The model under review builds one solid part; all positions refer to its coordinate system, in mm. Face numbers are marked on the shaded views. A direction names the side the tool comes from. Round coordinates to 2 decimals unless told otherwise and drop trailing zeros. Write each loop counter-clockwise with the first axis right and the second up, starting at its lowest first coordinate (ties: lowest second). Pieces come first, ordered by that corner, then holes. Notation, with made-up numbers: (-29, 80.5) -> (-2, 80.5) arc R32 ccw to (-2, 115.5) -> close; hole circle Ø11 at (68.5, 60). An arc over 180 degrees is marked (long way). Answer as a JSON object with one key per item and string values. Group by question number.
1) We need section D-D, the plane z = -6. Write out the cut boundary in (x, y), then the cut area to 3 significant figures.
2) We need section A-A, the plane x = 0. Write out the cut boundary in (y, z).
3) Mouldability with a two-part tool opening along Y and no side actions: class the marked faces 1, 2 and 3 as pulls with the +Y half, pulls with the -Y half, needs draft (parallel to the pull), parting line crosses it, or undercut.
4) To check wall thickness, follow probe 1 along X at (y, z) = (-1, -4.5); probe 2 along X at (y, z) = (-0.5, -2); probe 3 along Y at (x, z) = (1, -4.75). State the ranges of each line that lie inside material, in increasing order. Write a range as [from, to].
5) We need section B-B, the plane z = -12.5. Write out the cut boundary in (x, y), then the cut area to 3 significant figures.
6) We need section C-C, the plane z = -8.75. Write out the cut boundary in (x, y), then the cut area to 3 significant figures.
7) Machinability: for the marked faces 4, 5 and 6, which of the approach directions +Z, -Z, +X, -X, +Y, -Y give a long, thin tool a straight path to every point of the face, cutting with its end or side? Answer none if there is none.
8) Insertion check: pin 1 Ø1.5 at (y, z) = (0, -12.5) entering from -X; pin 2 Ø1.5 at (x, z) = (1, -7) entering from -Y; pin 3 Ø1 at (y, z) = (-1.5, -13.5) entering from -X. Each pin has a flat end and moves straight along its axis. Give the tip position at first contact, or say it passes through.
from build123d import *

# Parameters (mm, degrees)
F2_W          = 4.1
F2_H          = 8.2
F3_DEPTH      = 4.001
F3_DEPTH_BACK = 4.001
F5_D          = 3.3
F5_DEPTH      = 4.001
F6_D          = 2.5
F8_D          = 2.5


with BuildPart() as f1:
    # F0 (on Front) → F1 (revolve)
    with BuildSketch(Plane.XZ):
        Polygon((2.5, 0), (0, 0), (0, -16), (4, -16), (4, -7), (2.5, -1), align=None)
    revolve(axis=Axis((0, 0, -12.0333206053), (0, 0, -1)))

    # F2 (on Front) → F3 (cut, two sides)
    with BuildSketch(Plane.XZ) as f3_sk:
        with Locations((0, -11.9)):
            Rectangle(F2_W, F2_H)
    extrude(amount=F3_DEPTH, mode=Mode.SUBTRACT)
    extrude(f3_sk.sketch, amount=-F3_DEPTH_BACK, mode=Mode.SUBTRACT)

    # F5 (through all, one way)
    with BuildSketch(Plane(origin=(0, 0, 0), x_dir=(0, 1, 0), z_dir=(-1, 0, 0))):
        with Locations((0, 12.5)):
            Circle(F5_D / 2)
    extrude(amount=-F5_DEPTH, mode=Mode.SUBTRACT)

    # F6 (through all)
    with Locations(Plane.YZ):
        with Locations((0, -12.5)):
            Hole(F6_D / 2)

    # F8 (through all)
    with Locations(Plane.XY):
        with Locations((0, 0)):
            Hole(F8_D / 2)


solid = f1.part
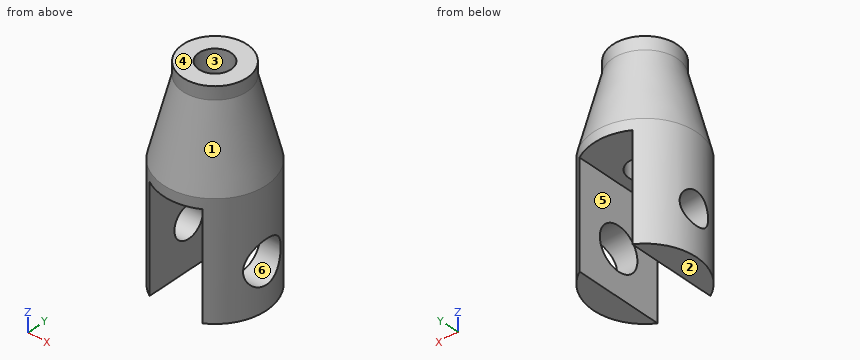
Here are the results:
{
 "1": {"outline": "circle Ø7.5 at (0, 0); hole circle Ø2.5 at (0, 0)", "area": "39.3 mm^2"},
 "2": {"outline": "(-4, -7.8) -> (-1.25, -7.8) -> (-1.25, 0) -> (-2.5, 0) -> (-2.5, -1) -> (-4, -7) -> close; (1.25, -7.8) -> (4, -7.8) -> (4, -7) -> (2.5, -1) -> (2.5, 0) -> (1.25, 0) -> close"},
 "3": {"face 1": "parting line crosses it", "face 2": "needs draft", "face 3": "undercut"},
 "4": {"probe 1": "x = [-3.22, -0.75], [0.75, 3.22]", "probe 2": "x = [-2.7, -1.15], [1.15, 2.7]", "probe 3": "y = [-3.29, -0.75], [0.75, 3.29]"},
 "5": {"outline": "(-3.8, -1.25) arc R4 ccw to (-2.05, -3.43) -> (-2.05, -1.25) -> close; (-3.8, 1.25) -> (-2.05, 1.25) -> (-2.05, 3.43) arc R4 ccw to start; (2.05, -3.43) arc R4 ccw to (3.64, -1.65) -> (2.05, -1.65) -> close; (2.05, 1.65) -> (3.64, 1.65) arc R4 ccw to (2.05, 3.43) -> close", "area": "8.20 mm^2"},
 "6": {"outline": "(-2.05, -3.43) -> (-2.05, 3.43) arc R4 ccw to start; (2.05, -3.43) arc R4 ccw to (2.05, 3.43) -> close", "area": "19.0 mm^2"},
 "7": {"face 4": "+Z, +X, -X, +Y, -Y", "face 5": "-Z, +Y, -Y", "face 6": "+X"},
 "8": {"pin 1": "passes through", "pin 2": "stops at y = -3.99", "pin 3": "stops at x = -3.87"}
}
